The model under review builds one solid part; all positions refer to its coordinate system, in mm. Face numbers are marked on the shaded views. A direction names the side the tool comes from. Round coordinates to 2 decimals unless told otherwise and drop trailing zeros. Order: outer loops, then holes, each group sorted by start corner. A loop starts at its lowest first (then second) coordinate and runs counter-clockwise, first axis right, second up.
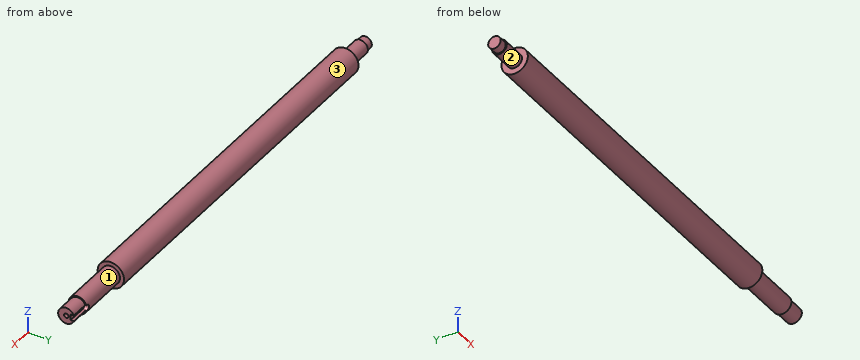
from build123d import *

# Parameters (mm, degrees)
CUT_EXTRUDE1_DEPTH = 14
SKETCH4_R          = 3
CUT_EXTRUDE2_DEPTH = 25


with BuildPart() as part:
    # Sketch1 → Revolve1 (revolve)
    with BuildSketch(Plane.XY):
        Polygon((254.240699987, 11), (279.240699987, 11), (279.240699987, 0), (-371.759300013, 0), (-371.759300013, 8.5), (-360.759300013, 8.5), (-360.759300013, 10), (-327.759300013, 10), (-327.759300013, 18), (182.240699987, 18), (182.240699987, 12.5), (254.240699987, 12.5), align=None)
    revolve(axis=Axis((279.240699987, 0, 0), (-1, 0, 0)))

    # Sketch3 → Cut-Extrude1 (cut)
    with BuildSketch(Plane(origin=(0, 20, 0), x_dir=(1, 0, 0), z_dir=(0, 1, 0))):
        with BuildLine():
            Line((279.240699987, -4), (253.217727507, -4))
            ThreePointArc((253.217727507, -4), (249.217727507, 0), (253.217727507, 4))
            Line((253.217727507, 4), (279.240699987, 4))
            ThreePointArc((279.240699987, 4), (283.240699987, 0), (279.240699987, -4))
        make_face()
    extrude(amount=-CUT_EXTRUDE1_DEPTH, mode=Mode.SUBTRACT)

    # Sketch4 → Cut-Extrude2 (cut)
    with BuildSketch(Plane(origin=(279.240699987, 0, 0), x_dir=(0, 0, -1), z_dir=(1, 0, 0))):
        with Locations(Location((0, 0, 0), (0, 0, 90))):
            Circle(SKETCH4_R)
    extrude(amount=-CUT_EXTRUDE2_DEPTH, mode=Mode.SUBTRACT)


solid = part.part
(1) Tool access review of the marked faces 1, 2 and 3: name each direction out of +Z, -Z, +X, -X, +Y, -Y from which nothing blocks a thin tool from reaching the whole face with its end or side.
(2) Clearance check with flat-ended pins moving along their axes: P1, Ø3, axis at y = 7, z = 12, coming from the -X side; P2, Ø12, axis at x = -209, z = 12.5, coming from the +Y side; P3, Ø1.8, axis at x = 269.5, y = 9, coming from the -Z side. State where each tip first meets the part, or that it passes through.
(3) We need section B-B (x = 201.5). Give the boundary of the cut face in (y, z), and give its area (3 significant figures).
(4) To check wall thickness, follow L1, parallel to Z at x = 259.5, y = 0; L2, parallel to X at y = -8.5, z = 1; L3, parallel to X at y = -10.5, z = 13. State the ranges of each line that lie inside material, in increasing order.
(5) We need section A-A (x = -7.5). Give the boundary of the cut face in (y, z), and give its area (3 significant figures).
Verdict:
1. face 1: +X
1. face 2: -X
1. face 3: +X, -X
2. P1: stops at x = -327.76
2. P2: stops at y = 16.79
2. P3: stops at z = -7.44
3. outline: circle Ø25 at (0, 0)
3. area: 491 mm2
4. L1: z = -11 to -3, 3 to 11
4. L2: x = -360.76 to 279.24
4. L3: x = -327.76 to 182.24
5. outline: circle Ø36 at (0, 0)
5. area: 1,020 mm2
